Input: part model. Units: mm. Frame: model coordinates. Face numbers are marked on the shaded views. Coordinates: 2 decimals unless noted, no trailing zeros. Order: outer loops, then holes, each group sorted by start corner. A loop starts at its lowest first (then second) coordinate and runs counter-clockwise, first axis right, second up. Notation, with made-up numbers: (18, 71.25) -> (40, 71.25) arc R11 cw to (40, 92.25) -> close; hole circle Ø3 at (58.5, 77). An arc over 180 degrees is marked (long way). Use one line per item in the form item = value. Start each with the question number.
1) Ray query, line 1 along Z through (x, y) = (0, 8); line 2 along X through (y, z) = (8, 0); line 3 along X through (y, z) = (12.5, 6). Return the intervals inside material, ascending.
2) Pin query (flat end, axial travel): pin 1 (8 mm diameter, centred on y = 14.5, z = -7, fed in from +X); pin 2 (1.5 mm diameter, centred on y = 3.5, z = -11.5, fed in from -X); pin 3 (5 mm diameter, centred on y = 10.5, z = 10, fed in from -X). Return the tip coordinate at first contact, or that it passes through.
3) Draft query along Z for the marked faces 1, 2 and 3. Return one class per face: pulls with the +Z half, pulls with the -Z half, needs draft (parallel to the pull), parting line crosses it, or undercut.
4) Section query A-A on y = 3.5. Output: boundary loops of the cut face in (x, z), then the cut area to 3 significant figures.
from build123d import *

# Parameters (mm, degrees)
BOSS_EXTRUDE1_DEPTH = 20
SKETCH2_OUTSIDE_W   = 116.37
SKETCH2_OUTSIDE_H   = 111.68
SKETCH2_OUTSIDE_R   = 15.155444566
CUT_EXTRUDE1_DEPTH  = 20
CUT_EXTRUDE1_TAPER  = 60
SKETCH3_R           = 13
CUT_EXTRUDE2_DEPTH  = 21


with BuildPart() as part:
    # Sketch1 → Boss-Extrude1 (new body)
    with BuildSketch(Plane(origin=(0, 0, 0), x_dir=(1, 0, 0), z_dir=(0, 1, 0))):
        Polygon((17.5, 0), (8.75, 15.155444566), (-8.75, 15.155444566), (-17.5, 0), (-8.75, -15.155444566), (8.75, -15.155444566), align=None)
    extrude(amount=BOSS_EXTRUDE1_DEPTH)

    # Sketch2 outside → Cut-Extrude1 (cut)
    with BuildSketch(Plane(origin=(0, 20, 0), x_dir=(1, 0, 0), z_dir=(0, 1, 0))):
        Rectangle(SKETCH2_OUTSIDE_W, SKETCH2_OUTSIDE_H)
        Circle(SKETCH2_OUTSIDE_R, mode=Mode.SUBTRACT)
    extrude(amount=-CUT_EXTRUDE1_DEPTH, taper=CUT_EXTRUDE1_TAPER, mode=Mode.SUBTRACT)

    # Sketch3 → Cut-Extrude2 (cut, through all)
    with BuildSketch(Plane(origin=(0, 20, 0), x_dir=(1, 0, 0), z_dir=(0, 1, 0))):
        Circle(SKETCH3_R)
    extrude(amount=-CUT_EXTRUDE2_DEPTH, mode=Mode.SUBTRACT)


solid = part.part
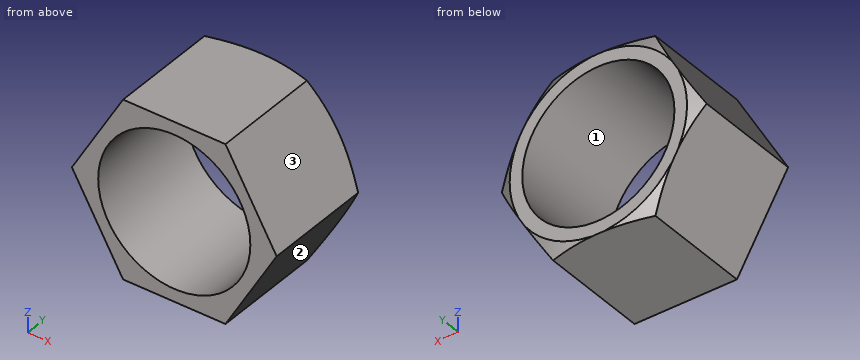
Answers below:
q1.line_1 = -15.16 to -13, 13 to 15.16
q1.line_2 = -17.5 to -13, 13 to 17.5
q1.line_3 = -14.04 to -11.53, 11.53 to 14.04
q2.pin_1 = 15.77
q2.pin_2 = -11.29
q2.pin_3 = -13.17
q3.face_1 = undercut
q3.face_2 = pulls with the -Z half
q3.face_3 = pulls with the +Z half
q4.outline = (-17.5, 0) -> (-8.75, -15.16) -> (8.75, -15.16) -> (17.5, 0) -> (8.75, 15.16) -> (-8.75, 15.16) -> close; hole circle Ø26 at (0, 0)
q4.area = 265 mm^2
